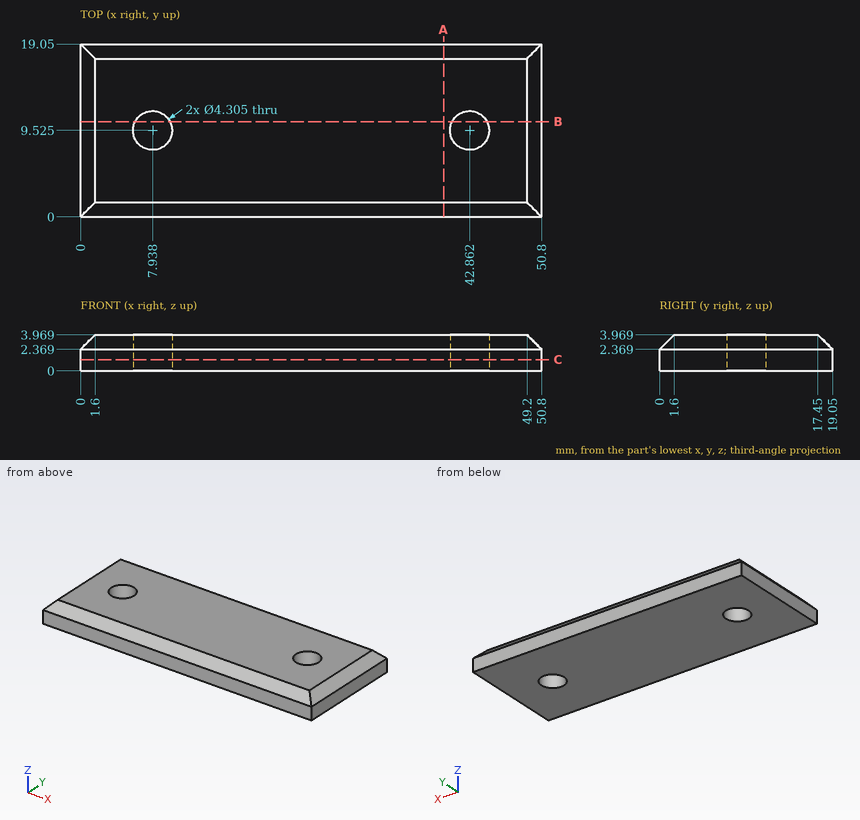
Source: three-view drawing plus pictorial views. Frame: mm from the lowest corner of the part. Round coordinates to 2 decimals unless told otherwise and drop trailing zeros. Loops run counter-clockwise (first coordinate to the right, second up) from the corner with the lowest first, then second, coordinate; pieces in that order, holes last. Notation, with made-up numbers: M 22.5,45.25 L 29.5,45.25 A13 cw 29.5,60.25 Z; hole C -12.75,81.5 d11. An arc over 180 degrees is marked long. Answer as CSV lines item,"result".
Q1. Cut plane B-B (y = 10.5). Return the cut outline in (x, z).
Verdict:
outline,"M 0,0 L 6.02,0 L 6.02,3.97 L 1.6,3.97 L 0,2.37 Z; M 9.86,0 L 40.94,0 L 40.94,3.97 L 9.86,3.97 Z; M 44.78,0 L 50.8,0 L 50.8,2.37 L 49.2,3.97 L 44.78,3.97 Z"
Q2. Cut plane A-A (x = 40). Return the cut outline in (y, z).
Verdict:
outline,"M 0,0 L 19.05,0 L 19.05,2.37 L 17.45,3.97 L 1.6,3.97 L 0,2.37 Z"
Q3. Cut plane C-C (z = 1.25). Count the separate pieces of the cut face and the enclosed holes in it.
Verdict:
separate pieces,"1"
enclosed holes,"2"
Q4. Line query: line 1 along X through (y, z) = (9.75, 1.65); line 2 along Y through (x, z) = (46, 3.55); line 3 along Y through (x, z) = (48, 3.3). Output: solid intervals per line, ascending.
Verdict:
line 1,"x = 0 to 5.8, 10.08 to 40.72, 45 to 50.8"
line 2,"y = 1.18 to 17.87"
line 3,"y = 0.93 to 18.12"
